```python
from build123d import *

# Parameters (mm, degrees)
F1_DEPTH = 127
F2_R     = 5.08
F3_SIZE  = 5.08
F4_R     = 2.5527
F5_DEPTH = 304.801


with BuildPart() as f1:
    # F0 (on Front) → F1 (new body)
    with BuildSketch(Plane.XZ):
        Polygon((-304.8, 0), (0, 0), (0, 38.1), (-6.35, 38.1), (-6.35, 6.35), (-298.45, 6.35), (-298.45, 38.1), (-304.8, 38.1), align=None)
    extrude(amount=-F1_DEPTH)

    # F2
    f2_edges = [f1.edges().sort_by_distance(p)[0] for p in [
        (-304.8, 63.5, 0),
        (0, 63.5, 0),
    ]]
    fillet(f2_edges, radius=F2_R)

    # F3
    f3_edges = [f1.edges().sort_by_distance(p)[0] for p in [
        (-152.4, 0, 6.35),
    ]]
    chamfer(f3_edges, length=F3_SIZE)

    # F4 (on Right) → F5 (cut, through all)
    with BuildSketch(Plane.YZ):
        with Locations((12.7, 12.7)):
            Circle(F4_R)
        with Locations((12.7, 25.4)):
            Circle(F4_R)
        with Locations((25.4, 25.4)):
            Circle(F4_R)
        with Locations((25.4, 12.7)):
            Circle(F4_R)
        with Locations((88.9, 12.7)):
            Circle(F4_R)
        with Locations((101.6, 12.7)):
            Circle(F4_R)
        with Locations((101.6, 25.4)):
            Circle(F4_R)
        with Locations((88.9, 25.4)):
            Circle(F4_R)
    extrude(amount=-F5_DEPTH, mode=Mode.SUBTRACT)


solid = f1.part
```
Work out the finished part from the listing and answer in its coordinate system (mm). Round coordinates to 2 decimals unless told otherwise and drop trailing zeros. Write each loop counter-clockwise with the first axis right and the second up, starting at its lowest first coordinate (ties: lowest second). Pieces come first, ordered by that corner, then holes. Notation, with made-up numbers: (-31.75, -20.5) -> (12.25, -20.5) arc R16 ccw to (12.25, 1.5) -> close; hole circle Ø8 at (69.5, -3.75). An arc over 180 degrees is marked (long way). Write each question's results on one line, items separated by ' | '.
1) Consider line 1 along Y through (x, z) = (-300, 25); line 2 along X through (y, z) = (100.5, 21); line 3 along Z through (x, y) = (-4.25, 101.6). Determine where each line is inside the solid, lowest interval first. Write a range as [from, to].
Findings:
line 1: y = [0, 10.18], [15.22, 22.88], [27.92, 86.38], [91.42, 99.08], [104.12, 127] | line 2: x = [-304.8, -298.45], [-6.35, 0] | line 3: z = [0.07, 10.15], [15.25, 22.85], [27.95, 38.1]
2) For a pull along Z with two mould halves and no side action, classify faces 1 (the cylindrical face through (-1.528, 64.389, 1.449)), 2 (the flat face through (-150, 65, 6.35)), 3 (the cylindrical face through (-3.131, 103.958, 11.722)), 4 (the flat face through (-304.8, 63, 22)) as +Z half, -Z half, draft (parallel to the pull), parting line (faces both ways), or undercut.
Findings:
face 1: -Z half | face 2: +Z half | face 3: undercut | face 4: draft
3) The part is cut by section A-A (y = 66). Write down the section's boundary in (x, z), and give its area (3 significant figures).
Findings:
outline: (-304.8, 5.08) arc R5.08 ccw to (-299.72, 0) -> (-5.08, 0) arc R5.08 ccw to (0, 5.08) -> (0, 38.1) -> (-6.35, 38.1) -> (-6.35, 6.35) -> (-298.45, 6.35) -> (-298.45, 38.1) -> (-304.8, 38.1) -> close | area: 2,330 mm²
4) The part is cut by section B-B (x = -179.5). Write down the section's boundary in (y, z), and give its area (3 significant figures).
Findings:
outline: (0, 0) -> (127, 0) -> (127, 6.35) -> (5.08, 6.35) -> (0, 1.27) -> close | area: 794 mm²
5) Flat-ended cylindrical pins translate along their axes: pin 1 (4.5 mm diameter, centred on y = 25.4, z = 25.4, fed in from +X); pin 2 (6.5 mm diameter, centred on y = 12.7, z = 25.4, fed in from -X); pin 3 (1.5 mm diameter, centred on x = -192.5, y = 29, fed in from +Z). Find the tip coordinate at first contact, or state that the pin passes through.
Findings:
pin 1: passes through | pin 2: stops at x = -304.8 | pin 3: stops at z = 6.35
